Design review of the part built by this model. Coordinates are the model's own, in mm. A direction names the side the tool comes from. Coordinates: 2 decimals unless noted, no trailing zeros. Write each loop counter-clockwise with the first axis right and the second up, starting at its lowest first coordinate (ties: lowest second). Pieces come first, ordered by that corner, then holes.
Q1. Add section A-A, the plane z = 14. Give the number of separate pieces and of enclosed holes in the cut face, plus the area to 3 significant figures.
Q2. Clearance check with flat-ended pins moving along their axes: pin 1 Ø1.5 at (x, y) = (14, -26) entering from +Z; pin 2 Ø1.9 at (x, z) = (4, -21) entering from -Y; pin 3 Ø7.5 at (x, y) = (0, -19.05) entering from +Z; pin 4 Ø3 at (y, z) = (4, 17) entering from +X. State where each tip first meets the part, or that it passes through.
Q3. Add section C-C, the plane y = -36.83. Give the boundary of the cut face in (x, z).
Q4. The part is to be moulded in two halves that separate along Y. For faces 1 (the face through (15, 0, 0)), 2 (the face through (-0.62, -32.11, 0.25)), 3 (the face through (0, 0, 21)), 4 (the face through (12.7, 37, 11)), say which applies: +Y half, -Y half, draft (parallel to the pull), parting line (faces both ways), or undercut.
Q5. Machinability: for faces 5 (the face through (0, -73.596, 0)), 6 (the face through (0, 23, 24.13)), 7 (the face through (-15, 0, 0)), 8 (the face through (0, -44, -17.78)), 9 (the face through (0, -44, 17.78)), which of the approach directions +Z, -Z, +X, -X, +Y, -Y give a long, thin tool a straight path to every point of the face, cutting with its end or side? Answer none if there is none.
Q6. To check wall thickness, follow probe 1 along X at (y, z) = (-19, -7); probe 2 along Y at (x, z) = (0, 8); probe 3 along Y at (x, z) = (0, 2). State the ranges of each line that lie inside material, in increasing order.
from build123d import *

# Parameters (mm, degrees)
SKETCH1_W           = 35.56
SKETCH1_H           = 35.56
BOSS_EXTRUDE1_DEPTH = 73.5965
SKETCH2_R           = 4.7625
CUT_EXTRUDE1_DEPTH  = 84.648591215
SKETCH3_W           = 25.4
SKETCH3_H           = 35.56
BOSS_EXTRUDE2_DEPTH = 44.45
SKETCH5_W           = 25.4
SKETCH5_H           = 44.45
BOSS_EXTRUDE3_DEPTH = 6.35
SKETCH6_W           = 25.4
SKETCH6_H           = 44.45
BOSS_EXTRUDE4_DEPTH = 6.35
SKETCH4_R           = 17.500000052
CUT_EXTRUDE2_DEPTH  = 84.232998938


with BuildPart() as part:
    # Sketch1 → Boss-Extrude1 (new body)
    with BuildSketch(Plane(origin=(0, 0, 0), x_dir=(1, 0, 0), z_dir=(0, 1, 0))):
        Rectangle(SKETCH1_W, SKETCH1_H)
    extrude(amount=-BOSS_EXTRUDE1_DEPTH)

    # Sketch2 → Cut-Extrude1 (cut, through all)
    with BuildSketch(Plane.XY.offset(17.78)):
        with Locations((0, -19.05)):
            Circle(SKETCH2_R)
        with Locations((0, -36.83)):
            Circle(SKETCH2_R)
        with Locations((0, -55.88)):
            Circle(SKETCH2_R)
    extrude(amount=-CUT_EXTRUDE1_DEPTH, mode=Mode.SUBTRACT)

    # Sketch3 → Boss-Extrude2 (add)
    with BuildSketch(Plane(origin=(0, 0, 0), x_dir=(1, 0, 0), z_dir=(0, 1, 0))):
        Rectangle(SKETCH3_W, SKETCH3_H)
    extrude(amount=BOSS_EXTRUDE2_DEPTH)

    # Sketch5 → Boss-Extrude3 (add)
    with BuildSketch(Plane.XY.offset(17.78)):
        with Locations((0, 22.225)):
            Rectangle(SKETCH5_W, SKETCH5_H)
    extrude(amount=BOSS_EXTRUDE3_DEPTH)

    # Sketch6 → Boss-Extrude4 (add)
    with BuildSketch(Plane(origin=(0, 0, -17.78), x_dir=(-1, 0, 0), z_dir=(0, 0, -1))):
        with Locations((0, 22.225)):
            Rectangle(SKETCH6_W, SKETCH6_H)
    extrude(amount=BOSS_EXTRUDE4_DEPTH)

    # Sketch4 → Cut-Extrude2 (cut, through all)
    with BuildSketch(Plane(origin=(12.7, 0, 0), x_dir=(0, 0, -1), z_dir=(1, 0, 0))):
        with Locations((0, 22.225)):
            Circle(SKETCH4_R)
    extrude(amount=-CUT_EXTRUDE2_DEPTH, mode=Mode.SUBTRACT)


solid = part.part
Here are the results:
1. separate pieces: 2
1. enclosed holes: 3
1. area: 3,000 mm2
2. pin 1: stops at z = 17.78
2. pin 2: stops at y = 0
2. pin 3: passes through
2. pin 4: stops at x = 12.7
3. outline: (-17.78, -17.78) - (-4.76, -17.78) - (-4.76, 17.78) - (-17.78, 17.78) - close; (4.76, -17.78) - (17.78, -17.78) - (17.78, 17.78) - (4.76, 17.78) - close
4. face 1: +Y half
4. face 2: undercut
4. face 3: -Y half
4. face 4: draft
5. face 5: +Z, -Z, +X, -X, -Y
5. face 6: +Z, +X, -X, +Y, -Y
5. face 7: +Z, -Z, -X, +Y
5. face 8: -Z, +X, -X, -Y
5. face 9: +Z, +X, -X, -Y
6. probe 1: x = -17.78 to -4.76, 4.76 to 17.78
6. probe 2: y = -73.6 to -60.64, -51.12 to -41.59, -32.07 to -23.81, -14.29 to 6.66, 37.79 to 44.45
6. probe 3: y = -73.6 to -60.64, -51.12 to -41.59, -32.07 to -23.81, -14.29 to 4.84, 39.61 to 44.45
